```python
from build123d import *

# Parameters (mm, degrees)
F0_W     = 42.3
F0_H     = 42.3
F0_R     = 1.5
F0_R_2   = 11
F1_DEPTH = 6.5
F2_W     = 42.3
F2_H     = 38
F3_DEPTH = 4
F6_DEPTH = 4
F7_DEPTH = 4
F8_DEPTH = 0.5
F9_DEPTH = 0.5


with BuildPart() as f1:
    # F0 (on Top) → F1 (new body)
    with BuildSketch(Plane.XY):
        with Locations((0.9411764706, -0.8529411765)):
            Rectangle(F0_W, F0_H)
        with Locations((-14.3088235294, -16.1029411765)):
            Circle(F0_R, mode=Mode.SUBTRACT)
        with Locations((0.6911764706, -1.1029411765)):
            Circle(F0_R_2, mode=Mode.SUBTRACT)
        with Locations((16.1911764706, -16.1029411765)):
            Circle(F0_R, mode=Mode.SUBTRACT)
        with Locations((-14.3088235294, 14.3970588235)):
            Circle(F0_R, mode=Mode.SUBTRACT)
        with Locations((16.1911764706, 14.3970588235)):
            Circle(F0_R, mode=Mode.SUBTRACT)
    extrude(amount=F1_DEPTH)

    # F2 (on face) → F3 (join)
    with BuildSketch(Plane(origin=(-20.2088235294, 0, 0), x_dir=(0, -1, 0), z_dir=(-1, 0, 0))):
        with Locations((0.8529411765, -12.5)):
            Rectangle(F2_W, F2_H)
    extrude(amount=F3_DEPTH)

    # F5 (on face) → F6 (join)
    with BuildSketch(Plane(origin=(0, 20.2970588235, 0), x_dir=(-1, 0, 0), z_dir=(0, 1, 0))):
        with BuildLine():
            ThreePointArc((-22.0911764706, 0), (3.080762749, -10.3491101908), (20.2088235294, -31.5))
            Line((20.2088235294, -31.5), (20.2088235294, 0))
            Line((20.2088235294, 0), (-22.0911764706, 0))
        make_face()
        Polygon((20.2088235294, 0), (20.2088235294, -31.5), (24.2088235294, -31.5), (24.2088235294, 6.5), (-22.0911764706, 6.5), (-22.0911764706, 0), align=None)
    extrude(amount=F6_DEPTH)

    # F4 (on face) → F7 (join)
    with BuildSketch(Plane.XZ.offset(22.0029411765)):
        with BuildLine():
            ThreePointArc((-20.2088235294, -31.5), (-3.080762749, -10.3491101908), (22.0911764706, 0))
            Line((22.0911764706, 0), (-20.2088235294, 0))
            Line((-20.2088235294, 0), (-20.2088235294, -31.5))
        make_face()
        Polygon((-20.2088235294, 0), (22.0911764706, 0), (22.0911764706, 6.5), (-24.2088235294, 6.5), (-24.2088235294, -31.5), (-20.2088235294, -31.5), align=None)
    extrude(amount=F7_DEPTH)

    # F8 (cut): a face of the model
    f8_faces = [f1.faces().sort_by_distance(p)[0] for p in [
        (-9.1642811897, -22.0029411765, -8.7688606087),
    ]]
    extrude(f8_faces, amount=-F8_DEPTH, mode=Mode.SUBTRACT)

    # F9 (cut): a face of the model
    f9_faces = [f1.faces().sort_by_distance(p)[0] for p in [
        (-9.1642811897, 20.2970588235, -8.7688606087),
    ]]
    extrude(f9_faces, amount=-F9_DEPTH, mode=Mode.SUBTRACT)


solid = f1.part
```
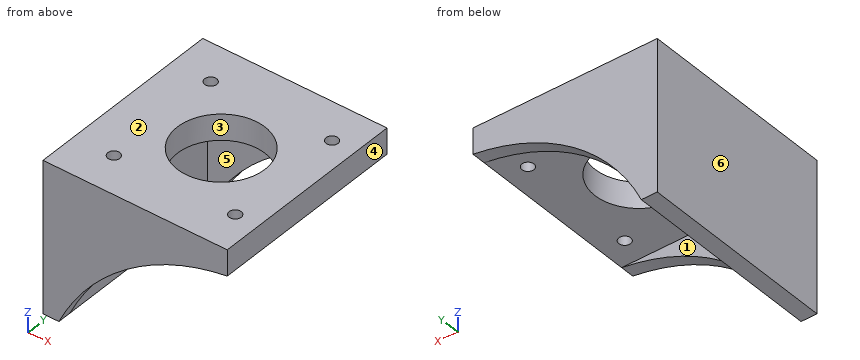
Verification items for the finished model (mm, model axes). Face numbers are marked on the shaded views. A direction names the side the tool comes from. Give positions to 0.01 mm unless a question says otherwise; leave off trailing zeros. Loops run counter-clockwise (first coordinate to the right, second up) from the corner with the lowest first, then second, coordinate; pieces in that order, holes last.
1. Section check B-B, the plane x = -2. Enter the section's corners in (y, z).
2. Set-up check for the marked faces 1 and 2: record each of +Z, -Z, +X, -X, +Y, -Y from which the full face is reachable in a straight line by a thin tool's end or side.
3. Mould release check, pull along X, two halves, no side actions. Record for the marked faces 3, 4, 5 and 6: released by +X, released by -X, zero draft, split by the parting line, or undercut.
4. Section check A-A, the plane y = 1. Enter the section's corners in (x, z).
5. Go/stop test with flat-tipped pins: pin 1 Ø4 at (x, y) = (-14.31, -16.1) entering from -Z; pin 2 Ø3 at (y, z) = (-11.5, -9.5) entering from +X. Record where each tip stops, or that it passes through.
6. Thickness scan on line 1 (Y direction, x = -18.5, z = -20); line 2 (Z direction, x = -13.5, y = 17.5); line 3 (X direction, y = 16, z = -15). Record the ranges inside material, lowest first.
7. Section check C-C, the plane y = 19.5. Enter the section's corners in (x, z).
8. Section check D-D, the plane z = -7. Enter the section's corners in (x, y).
Geometry says:
1. outline: (-26, -9.56) - (-22.5, -9.56) - (-22.5, 0) - (-11.77, 0) - (-11.77, 6.5) - (-26, 6.5) - close; (9.56, 0) - (20.8, 0) - (20.8, -9.56) - (24.3, -9.56) - (24.3, 6.5) - (9.56, 6.5) - close
2. face 1: -Z, +X
2. face 2: +Z, +X, -X, +Y, -Y
3. face 3: undercut
3. face 4: released by +X
3. face 5: zero draft
3. face 6: released by -X
4. outline: (-24.21, -31.5) - (-20.21, -31.5) - (-20.21, 0) - (-10.11, 0) - (-10.11, 6.5) - (-24.21, 6.5) - close; (11.49, 0) - (22.09, 0) - (22.09, 6.5) - (11.49, 6.5) - close
5. pin 1: stops at z = 0
5. pin 2: stops at x = -20.21
6. line 1: y = -26 to -22.5, 20.8 to 24.3
6. line 2: z = 0 to 6.5
6. line 3: x = -24.21 to -20.21
7. outline: (-24.21, -31.5) - (-20.21, -31.5) - (-20.21, 0) - (22.09, 0) - (22.09, 6.5) - (-24.21, 6.5) - close
8. outline: (-24.21, -26) - (1.98, -26) - (1.98, -22.5) - (-20.21, -22.5) - (-20.21, 20.8) - (1.98, 20.8) - (1.98, 24.3) - (-24.21, 24.3) - close
